Here's the drawing with two shaded views (mm, measured from the low corner). I have some questions. Give positions to 0.01 mm unless a question says otherwise; leave off trailing zeros. Loops run counter-clockwise (first coordinate to the right, second up) from the corner with the lowest first, then second, coordinate; pieces in that order, holes last. Notation, with made-up numbers: (45.5, -9) -> (97.5, -9) arc R11 cw to (97.5, 9) -> close; hole circle Ø6 at (19, 68). An arc over 180 degrees is marked (long way). Put each result on its own line as item: value.
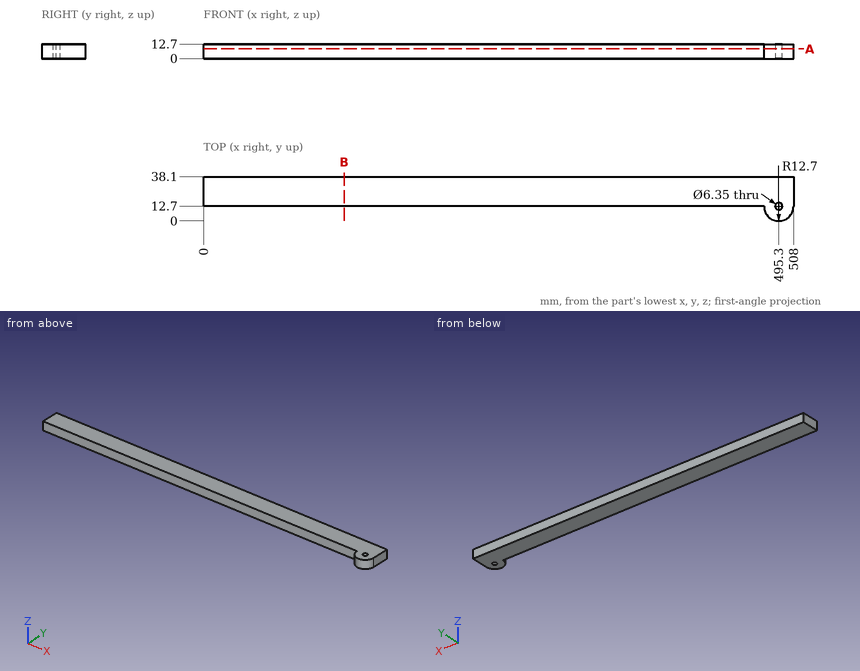
1. I need wall thicknesses on line 1 (Y direction, x = 495.3, z = 5.75) (3 decimals); line 2 (Y direction, x = 314, z = 1.5); line 3 (X direction, y = 10, z = 11). Which ranges of each line are inside material? Lowest first, please.
Recorded:
line 1: y = 0 to 9.525, 15.875 to 38.1
line 2: y = 12.7 to 38.1
line 3: x = 482.89 to 493.63, 496.97 to 507.71
2. If we section it at B-B (x = 121): List the corners of the cut face in (y, z) for me.
Recorded:
outline: (12.7, 0) -> (38.1, 0) -> (38.1, 12.7) -> (12.7, 12.7) -> close
3. If we section it at A-A (z = 8.5): List the corners of the cut face in (x, y) for me (3 decimals).
Recorded:
outline: (0, 12.7) -> (482.6, 12.7) arc R12.7 ccw to (508, 12.7) -> (508, 38.1) -> (0, 38.1) -> close; hole circle Ø6.35 at (495.3, 12.7)
4. I'm going to push a flat-ended pin straight in: pin 1 (6 mm diameter, centred on x = 429, z = 10.5, fed in from -Y). Where does the tip first touch, or does it pass through?
Recorded:
pin 1: stops at y = 12.7
